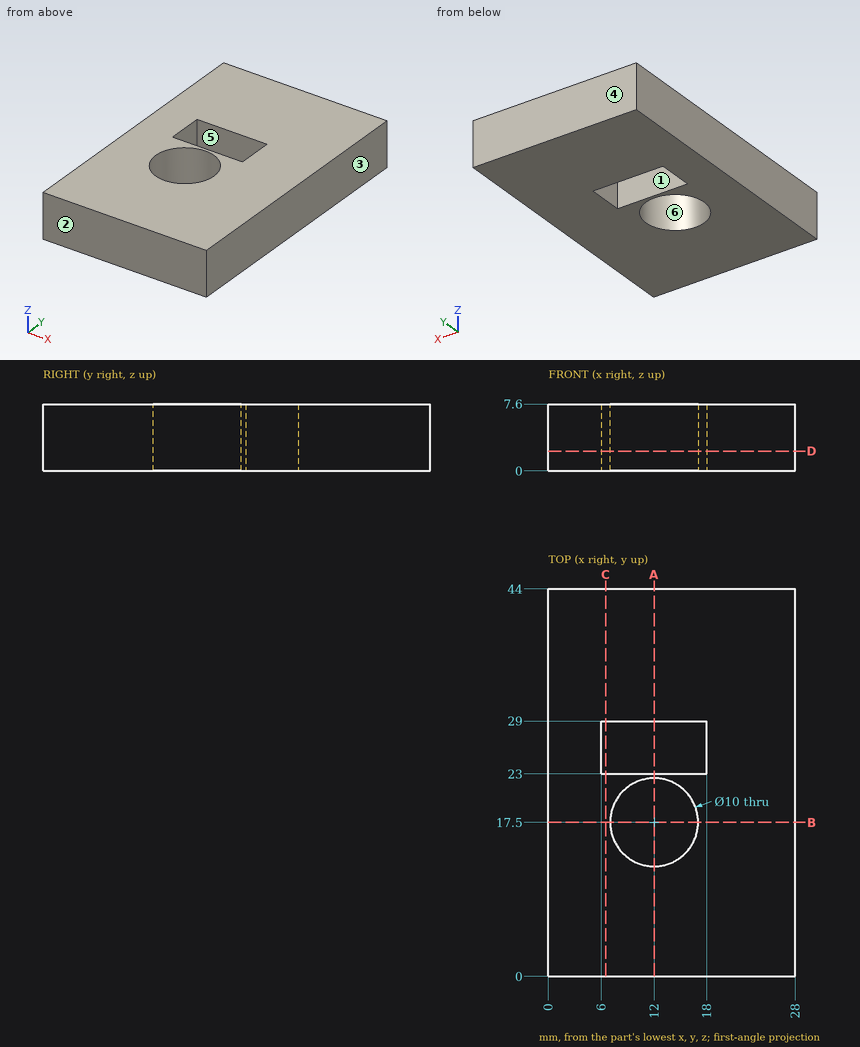
Geometry: see drawing. Coordinates: mm, zero at the bounding-box minimum. A direction names the side the tool comes from. Give positions to 0.01 mm unless a question says otherwise; leave off trailing zeros. Loops run counter-clockwise (first coordinate to the right, second up) from the corner with the lowest first, then second, coordinate; pieces in that order, holes last. Notation, with made-up numbers: (-11, 35.25) -> (18, 35.25) arc R19 cw to (18, 54.25) -> close; hole circle Ø7 at (61, -26). An arc over 180 degrees is marked (long way). Put each result on its own line as item: value.
1. Ray query, line 1 along Y through (x, z) = (12, 5.5); line 2 along X through (y, z) = (21.5, 2.75). Return the intervals inside material, ascending. Write a range as [from, to].
Taken from the geometry:
line 1: y = [0, 12.5], [22.5, 23], [29, 44]
line 2: x = [0, 9], [15, 28]
2. Set-up query: the marked faces 1 and 2. Return all of +Z, -Z, +X, -X, +Y, -Y with unobstructed straight access to the full face (end or side cutting, diameter ignored); none if empty.
Taken from the geometry:
face 1: +Z, -Z
face 2: +Z, -Z, +X, -X, -Y
3. Pull-direction query (Y, two-part tool) for the marked faces 3, 4, 5 and 6; classes: released by +Y, released by -Y, zero draft, split by the parting line, or undercut.
Taken from the geometry:
face 3: zero draft
face 4: released by +Y
face 5: undercut
face 6: undercut
4. Cut plane A-A (x = 12). Return the cut outline in (y, z).
Taken from the geometry:
outline: (0, 0) -> (12.5, 0) -> (12.5, 7.6) -> (0, 7.6) -> close; (22.5, 0) -> (23, 0) -> (23, 7.6) -> (22.5, 7.6) -> close; (29, 0) -> (44, 0) -> (44, 7.6) -> (29, 7.6) -> close
5. Cut plane C-C (x = 6.5). Return the cut outline in (y, z), plus the area to 3 significant figures.
Taken from the geometry:
outline: (0, 0) -> (23, 0) -> (23, 7.6) -> (0, 7.6) -> close; (29, 0) -> (44, 0) -> (44, 7.6) -> (29, 7.6) -> close
area: 289 mm2
6. Cut plane B-B (y = 17.5). Return the cut outline in (x, z), plus the area to 3 significant figures.
Taken from the geometry:
outline: (0, 0) -> (7, 0) -> (7, 7.6) -> (0, 7.6) -> close; (17, 0) -> (28, 0) -> (28, 7.6) -> (17, 7.6) -> close
area: 137 mm2
7. Cut plane D-D (z = 2.25). Return the cut outline in (x, y).
Taken from the geometry:
outline: (0, 0) -> (28, 0) -> (28, 44) -> (0, 44) -> close; hole (6, 23) -> (18, 23) -> (18, 29) -> (6, 29) -> close; hole circle Ø10 at (12, 17.5)
